```python
from build123d import *

# Parameters (mm, degrees)
F1_DEPTH = 28.575
F2_R     = 1.5875
F2_R_2   = 1.6042654536
F3_DEPTH = 6.35


with BuildPart() as f1:
    # F0 (on Front) → F1 (new body, symmetric)
    with BuildSketch(Plane.XZ):
        with BuildLine():
            Line((24.765, 40.5231858473), (-26.035, 40.5231858473))
            ThreePointArc((-26.035, 40.5231858473), (-43.9955122421, 33.0836980894), (-51.435, 15.1231858473))
            Line((-51.435, 15.1231858473), (-51.435, -16.6268141527))
            Line((-51.435, -16.6268141527), (50.165, -16.6268141527))
            Line((50.165, -16.6268141527), (50.165, 15.1231858473))
            ThreePointArc((50.165, 15.1231858473), (42.7255122421, 33.0836980894), (24.765, 40.5231858473))
        make_face()
    extrude(amount=F1_DEPTH, both=True)

    # F2 (on face) → F3 (join)
    with BuildSketch(Plane.XZ.offset(28.575)):
        with BuildLine():
            ThreePointArc((-8.6864773719, -16.6268141527), (-7.4177420061, -13.5638160255), (-6.985, -10.2768141527))
            ThreePointArc((-6.985, -10.2768141527), (-22.9720018728, 1.9904438412), (-30.6835226281, -16.6268141527))
            Line((-30.6835226281, -16.6268141527), (-8.6864773719, -16.6268141527))
        make_face()
        with Locations((-19.685, -10.2768141527)):
            Circle(F2_R, mode=Mode.SUBTRACT)
        with BuildLine():
            Line((-8.6864773719, -16.6268141527), (-30.6835226281, -16.6268141527))
            ThreePointArc((-30.6835226281, -16.6268141527), (-19.685, -22.9768141527), (-8.6864773719, -16.6268141527))
        make_face()
        with BuildLine():
            Line((29.3535084774, -16.6268141527), (7.4764915226, -16.6268141527))
            ThreePointArc((7.4764915226, -16.6268141527), (18.415, -22.9248759691), (29.3535084774, -16.6268141527))
        make_face()
        with BuildLine():
            ThreePointArc((31.0630618164, -10.2768141527), (15.1269507068, 1.9363836086), (7.4764915226, -16.6268141527))
            Line((7.4764915226, -16.6268141527), (29.3535084774, -16.6268141527))
            ThreePointArc((29.3535084774, -16.6268141527), (30.6281977613, -13.5648634459), (31.0630618164, -10.2768141527))
        make_face()
        with Locations((18.415, -10.2768141527)):
            Circle(F2_R_2, mode=Mode.SUBTRACT)
    extrude(amount=F3_DEPTH)

    # F4: F1 across plane


with BuildPart() as f1_1:
    add(f1.part)
    add(f1.part.mirror(Plane.XZ))


solid = f1_1.part
```
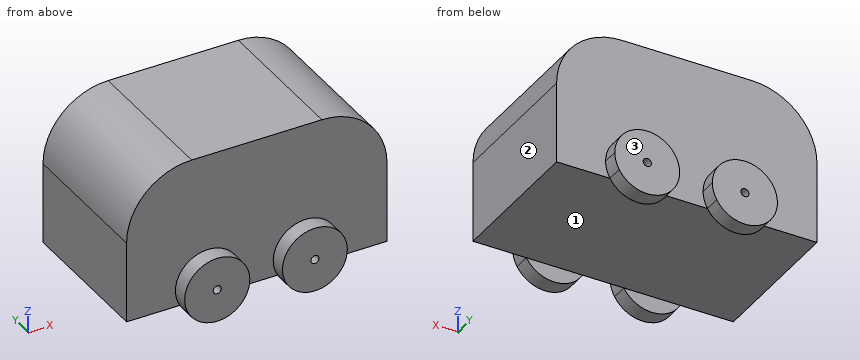
Read the model definition and answer for the solid it produces. Units are mm, in the model's axes. Face numbers are marked on the shaded views. Give positions to 0.01 mm unless a question says otherwise; leave off trailing zeros. Order: outer loops, then holes, each group sorted by start corner. A loop starts at its lowest first (then second) coordinate and runs counter-clockwise, first axis right, second up. Notation, with made-up numbers: (76, 2) -> (122, 2) arc R17 ccw to (122, 28) -> close; hole circle Ø8 at (51, 59). An arc over 180 degrees is marked (long way). Write item = value, one per line.
1. Given pin 1 (4 mm diameter, centred on x = -25.5, z = 9, fed in from -Y) (3 decimals); pin 2 (10 mm diameter, centred on x = -14.5, z = 10.5, fed in from +Y) (3 decimals); pin 3 (6 mm diameter, centred on x = 39, y = 5, fed in from +Z), each flat-ended and moving along its own axis, determine where each tip first touches the part or whether it passes through.
Numbers:
pin_1 = -28.575
pin_2 = 28.575
pin_3 = 37.9
2. The mould has two halves that part along Y. Classify the marked faces 1, 2 and 3: +Y half, -Y half, draft (parallel to the pull), parting line (faces both ways), or undercut.
Numbers:
face_1 = undercut
face_2 = draft
face_3 = +Y half
3. A cutting plane is placed at A-A, the plane y = -10. Write down the section's boundary in (x, z) (3 decimals), and give its area (3 significant figures).
Numbers:
outline = (-51.435, -16.627) -> (50.165, -16.627) -> (50.165, 15.123) arc R25.4 ccw to (24.765, 40.523) -> (-26.035, 40.523) arc R25.4 ccw to (-51.435, 15.123) -> close
area = 5,530 mm²
4. A cutting plane is placed at B-B, the plane x = 10. Write down the section's boundary in (y, z) (3 decimals).
Numbers:
outline = (-34.925, -19.719) -> (-28.575, -19.719) -> (-28.575, -16.627) -> (28.575, -16.627) -> (28.575, -19.719) -> (34.925, -19.719) -> (34.925, -0.834) -> (28.575, -0.834) -> (28.575, 40.523) -> (-28.575, 40.523) -> (-28.575, -0.834) -> (-34.925, -0.834) -> close
5. Straight lines are drawn through the part: line 1 along Y through (x, z) = (-12, 14) (3 decimals); line 2 along Z through (x, y) = (10, 0.5); line 3 along Z through (x, y) = (-19, -31.5). For each, find the intervals that lie inside material, in ascending order.
Numbers:
line_1 = -28.575 to 28.575
line_2 = -16.63 to 40.52
line_3 = -22.96 to -11.71, -8.84 to 2.4
6. A cutting plane is placed at C-C, the plane z = -1. Write down the section's boundary in (x, y) (3 decimals), and give its area (3 significant figures).
Numbers:
outline = (-51.435, -28.575) -> (-28.359, -28.575) -> (-28.359, -34.925) -> (-11.011, -34.925) -> (-11.011, -28.575) -> (9.818, -28.575) -> (9.818, -34.925) -> (27.012, -34.925) -> (27.012, -28.575) -> (50.165, -28.575) -> (50.165, 28.575) -> (27.012, 28.575) -> (27.012, 34.925) -> (9.818, 34.925) -> (9.818, 28.575) -> (-11.011, 28.575) -> (-11.011, 34.925) -> (-28.359, 34.925) -> (-28.359, 28.575) -> (-51.435, 28.575) -> close
area = 6,250 mm²
7. A cutting plane is placed at D-D, the plane x = -22.5. Write down the section's boundary in (y, z) (3 decimals).
Numbers:
outline = (-34.925, -22.661) -> (-28.575, -22.661) -> (-28.575, -16.627) -> (28.575, -16.627) -> (28.575, -22.661) -> (34.925, -22.661) -> (34.925, 2.107) -> (28.575, 2.107) -> (28.575, 40.523) -> (-28.575, 40.523) -> (-28.575, 2.107) -> (-34.925, 2.107) -> close
